```python
from build123d import *

# Parameters (mm, degrees)
SKETCH_1_W          = 80
SKETCH_1_H          = 80
SKETCH_1_R          = 2.65
SKETCH_1_R_2        = 1.6
SKETCH_1_R_3        = 18
EXTRUDE_1_DEPTH     = 4
SKETCH_2_R          = 1.55
CUT_EXTRUDE_1_DEPTH = 57.709787515
SKETCH_4_R          = 20
CUT_EXTRUDE_2_DEPTH = 57.709787515
SKETCH_5_W          = 141.692074253
SKETCH_5_H          = 118.011672495
CUT_EXTRUDE_3_DEPTH = 1


with BuildPart() as part:
    # 草图1 → 凸台-拉伸1 (new body)
    with BuildSketch(Plane.XY):
        Rectangle(SKETCH_1_W, SKETCH_1_H)
        with Locations((-32.5, 32.5)):
            Circle(SKETCH_1_R, mode=Mode.SUBTRACT)
        with Locations((-32.5, -32.5)):
            Circle(SKETCH_1_R, mode=Mode.SUBTRACT)
        with Locations((32.5, 32.5)):
            Circle(SKETCH_1_R_2, mode=Mode.SUBTRACT)
        with Locations((32.5, -32.5)):
            Circle(SKETCH_1_R_2, mode=Mode.SUBTRACT)
        Circle(SKETCH_1_R_3, mode=Mode.SUBTRACT)
    extrude(amount=EXTRUDE_1_DEPTH)

    # 草图2 → 切除-拉伸1 (cut, through all)
    with BuildSketch(Plane.XY.offset(4)):
        with Locations((-12.5, 21.650635095)):
            Circle(SKETCH_2_R)
        with Locations((12.5, 21.650635095)):
            Circle(SKETCH_2_R)
        with Locations((25, 0)):
            Circle(SKETCH_2_R)
        with Locations((12.5, -21.650635095)):
            Circle(SKETCH_2_R)
        with Locations((-12.5, -21.650635095)):
            Circle(SKETCH_2_R)
        with Locations((-25, 0)):
            Circle(SKETCH_2_R)
    extrude(amount=-CUT_EXTRUDE_1_DEPTH, mode=Mode.SUBTRACT)

    # 草图4 → 切除-拉伸2 (cut, through all)
    with BuildSketch(Plane(origin=(0, 0, 0), x_dir=(-1, 0, 0), z_dir=(0, 0, -1))):
        Circle(SKETCH_4_R)
    extrude(amount=-CUT_EXTRUDE_2_DEPTH, mode=Mode.SUBTRACT)

    # 草图5 → 切除-拉伸3 (cut)
    with BuildSketch(Plane(origin=(0, 0, 0), x_dir=(-1, 0, 0), z_dir=(0, 0, -1))):
        with Locations((12.88109766, -5.92010044)):
            Rectangle(SKETCH_5_W, SKETCH_5_H)
    extrude(amount=-CUT_EXTRUDE_3_DEPTH, mode=Mode.SUBTRACT)


solid = part.part
```
Here's how the part is built. I have some questions about the finished solid (model axes, mm). Give positions to 0.01 mm unless a question says otherwise; leave off trailing zeros. Write each loop counter-clockwise with the first axis right and the second up, starting at its lowest first coordinate (ties: lowest second). Pieces come first, ordered by that corner, then holes. Notation, with made-up numbers: (65.25, 13) -> (72.25, 13) arc R26 cw to (72.25, 48) -> close; hole circle Ø3 at (60.5, 73). An arc over 180 degrees is marked (long way). Write each question's results on one line, items separated by ' | '.
Item 1: Suppose I cut it at A-A on x = -32.5. Write out the boundary of the cut face in (y, z).
Output:
outline: (-40, 1) -> (-35.15, 1) -> (-35.15, 4) -> (-40, 4) -> close; (-29.85, 1) -> (29.85, 1) -> (29.85, 4) -> (-29.85, 4) -> close; (35.15, 1) -> (40, 1) -> (40, 4) -> (35.15, 4) -> close
Item 2: Suppose I cut it at C-C on x = 25. Write out the boundary of the cut face in (y, z), plus the area to 3 significant figures.
Output:
outline: (-40, 1) -> (-1.55, 1) -> (-1.55, 4) -> (-40, 4) -> close; (1.55, 1) -> (40, 1) -> (40, 4) -> (1.55, 4) -> close | area: 231 mm^2
Item 3: We'd pull the mould along Y, two halves only. Please class faces 1 (the face through (12.16, 20.14, 2.52)), 2 (the face through (40, -1, 2)), 3 (the face through (-1, 40, 2)): pulls with the +Y half, pulls with the -Y half, needs draft (parallel to the pull), parting line crosses it, or undercut.
Output:
face 1: undercut | face 2: needs draft | face 3: pulls with the +Y half
Item 4: Suppose I cut it at D-D on z = 1.45. Give the number of separate pieces and of enclosed holes in the cut face, plus the area to 3 significant figures.
Output:
separate pieces: 1 | enclosed holes: 11 | area: 5,040 mm^2
Item 5: Suppose I cut it at B-B on y = 32.5. Write out the boundary of the cut face in (x, z).
Output:
outline: (-40, 1) -> (-35.15, 1) -> (-35.15, 4) -> (-40, 4) -> close; (-29.85, 1) -> (30.9, 1) -> (30.9, 4) -> (-29.85, 4) -> close; (34.1, 1) -> (40, 1) -> (40, 4) -> (34.1, 4) -> close
Item 6: If I drill on L1, parallel to X at y = 32.5, z = 2.6; L2, parallel to Y at x = -32.5, z = 2.4; L3, parallel to Y at x = 12.5, z = 2.35, over which ranges is the centre line in solid material (lowest first)?
Output:
L1: x = -40 to -35.15, -29.85 to 30.9, 34.1 to 40 | L2: y = -40 to -35.15, -29.85 to 29.85, 35.15 to 40 | L3: y = -40 to -23.2, -20.1 to -15.61, 15.61 to 20.1, 23.2 to 40
